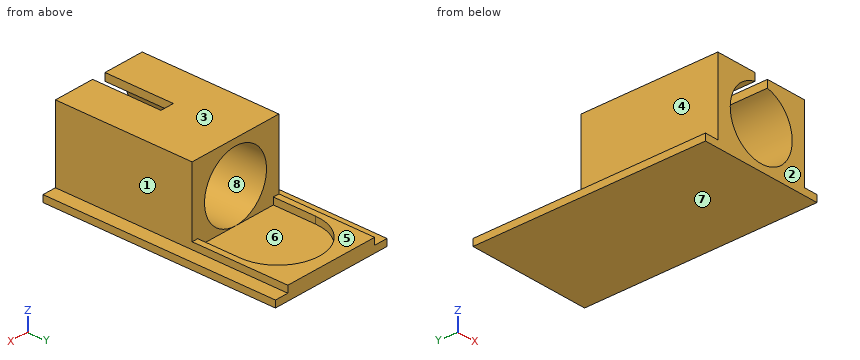
```python
from build123d import *

# Parameters (mm, degrees)
ESQUISSE1_W                  = 90
ESQUISSE1_H                  = 170
BOSS_EXTRU_1_DEPTH           = 5
ESQUISSE2_W                  = 70
ESQUISSE2_H                  = 100
BOSS_EXTRU_2_DEPTH           = 55
ENL_V_MAT_EXTRU_2_REACH      = 766.465
ESQUISSE4_R                  = 25
ENL_V_MAT_EXTRU_3_REACH      = 1014.096
ENL_V_MAT_EXTRU_3_END_RADIUS = 25
ESQUISSE5_W                  = 10
ESQUISSE5_H                  = 50
ESQUISSE6_W                  = 70
ESQUISSE6_H                  = 70
BOSS_EXTRU_3_DEPTH           = 5
ENL_V_MAT_EXTRU_4_DEPTH      = 5


with BuildPart() as part:
    # Esquisse1 → Boss.-Extru.1 (new body)
    with BuildSketch(Plane.XY):
        with Locations((-710.517990966, -585.769230769)):
            Rectangle(ESQUISSE1_W, ESQUISSE1_H)
    extrude(amount=BOSS_EXTRU_1_DEPTH)

    # Esquisse2 → Boss.-Extru.2 (add)
    with BuildSketch(Plane.XY.offset(5)):
        with Locations((-710.517990966, -620.769230769)):
            Rectangle(ESQUISSE2_W, ESQUISSE2_H)
    extrude(amount=BOSS_EXTRU_2_DEPTH)

    # Esquisse4 → Enlèv. mat.-Extru.2 (cut, up to next)
    with BuildSketch(Plane(origin=(0, -570.769230769, 0), x_dir=(1, 0, 0), z_dir=(0, 1, 0)), mode=Mode.PRIVATE) as enl_v_mat_extru_2_sk1:
        with Locations(Location((-710.517990966, -30, 0), (0, 0, 270))):
            Circle(ESQUISSE4_R)
    enl_v_mat_extru_2_tool1 = extrude(enl_v_mat_extru_2_sk1.sketch, amount=-ENL_V_MAT_EXTRU_2_REACH, mode=Mode.PRIVATE) & part.part
    add(enl_v_mat_extru_2_tool1.solids().sort_by_distance((-710.517991, -570.769231, 30))[0], mode=Mode.SUBTRACT)

    # Enlèv. mat.-Extru.3: up to this cylinder (the profile starts outside it)
    enl_v_mat_extru_3_end = Plane(origin=(-710.517990966, -645.769231, 30), z_dir=(0, 1, 0)) * Cylinder(ENL_V_MAT_EXTRU_3_END_RADIUS, 2079.192, mode=Mode.PRIVATE)
    # Esquisse5 → Enlèv. mat.-Extru.3 (cut, up to the surface)
    with BuildSketch(Plane.XY.offset(60), mode=Mode.PRIVATE) as enl_v_mat_extru_3_sk1:
        with Locations((-710.517990966, -645.769230769)):
            Rectangle(ESQUISSE5_W, ESQUISSE5_H)
    enl_v_mat_extru_3_tool1 = extrude(enl_v_mat_extru_3_sk1.sketch, amount=-ENL_V_MAT_EXTRU_3_REACH, mode=Mode.PRIVATE) - enl_v_mat_extru_3_end
    add(enl_v_mat_extru_3_tool1.solids().sort_by_distance((-710.517991, -645.769231, 60))[0], mode=Mode.SUBTRACT)

    # Esquisse6 → Boss.-Extru.3 (add)
    with BuildSketch(Plane.XY.offset(5)):
        with Locations((-710.517990966, -535.769230769)):
            Rectangle(ESQUISSE6_W, ESQUISSE6_H)
    extrude(amount=BOSS_EXTRU_3_DEPTH)

    # Esquisse7 → Enlèv. mat.-Extru.4 (cut)
    with BuildSketch(Plane.XY.offset(10)):
        with BuildLine():
            Line((-741.017990966, -539.769230769), (-741.017990966, -570.769230769))
            Line((-741.017990966, -570.769230769), (-680.017990966, -570.769230769))
            Line((-680.017990966, -570.769230769), (-680.017990966, -539.769230769))
            ThreePointArc((-680.017990966, -539.769230769), (-710.517990966, -509.269230769), (-741.017990966, -539.769230769))
        make_face()
    extrude(amount=-ENL_V_MAT_EXTRU_4_DEPTH, mode=Mode.SUBTRACT)


solid = part.part
```
Geometry check sheet. Reference: the model listing, model coordinates, mm. Face numbers are marked on the shaded views. A direction names the side the tool comes from. Coordinates: 2 decimals unless noted, no trailing zeros. Write each loop counter-clockwise with the first axis right and the second up, starting at its lowest first coordinate (ties: lowest second). Pieces come first, ordered by that corner, then holes. Notation, with made-up numbers: M -18.5,13.5 L -10.5,13.5 A13 cw -10.5,19.5 Z; hole C -4.75,25.5 d6. An arc over 180 degrees is marked long. Answer as a JSON object with one key per item and string values.
1. Scan lines: L1, parallel to X at y = -645, z = 30; L2, parallel to Y at x = -738.5, z = 50; L3, parallel to Y at x = -711, z = 8.5. Record each from-to range of solid material in increasing order.
Answers below:
{"L1": "x = -745.52 to -735.52, -685.52 to -675.52", "L2": "y = -670.77 to -570.77", "L3": "y = -509.27 to -500.77"}
2. Section check C-C, the plane y = -538. Enter the section's corners in (x, z).
Answers below:
{"outline": "M -755.52,0 L -665.52,0 L -665.52,5 L -675.52,5 L -675.52,10 L -680.07,10 L -680.07,5 L -740.97,5 L -740.97,10 L -745.52,10 L -745.52,5 L -755.52,5 Z"}
3. Section check B-B, the plane x = -700. Enter the section's corners in (y, z), plus the area to 3 significant figures.
Answers below:
{"outline": "M -670.77,0 L -500.77,0 L -500.77,10 L -511.14,10 L -511.14,5 L -570.77,5 L -570.77,7.32 L -670.77,7.32 Z; M -670.77,52.68 L -570.77,52.68 L -570.77,60 L -670.77,60 Z", "area": "1,870 mm²"}
4. Section check D-D, the plane x = -712.5. Enter the section's corners in (y, z).
Answers below:
{"outline": "M -670.77,0 L -500.77,0 L -500.77,10 L -509.33,10 L -509.33,5 L -570.77,5 L -570.77,5.08 L -670.77,5.08 Z; M -620.77,54.92 L -570.77,54.92 L -570.77,60 L -620.77,60 Z"}
5. Tool access check on the marked faces 1, 2, 3, 4 and 5. Record the directions out of +Z, -Z, +X, -X, +Y, -Y that give a thin tool (end or side, any length) a straight path to the whole face; none if there is none.
Answers below:
{"face 1": "+Z, +X, +Y, -Y", "face 2": "+Z, -Z, +X, -X, -Y", "face 3": "+Z, +X, -X, +Y, -Y", "face 4": "+Z, -X, +Y, -Y", "face 5": "+Z, +X, -X, +Y"}
6. Go/stop test with flat-tipped pins: pin 1 Ø4 at (y, z) = (-549, 7.5) entering from -X; pin 2 Ø1 at (y, z) = (-567.5, 9.5) entering from +X; pin 3 Ø5 at (x, y) = (-752, -614.5) entering from +Z. Record where each tip stops, or that it passes through.
Answers below:
{"pin 1": "stops at x = -745.52", "pin 2": "stops at x = -675.52", "pin 3": "stops at z = 5"}
7. Draft check along Z on the marked faces 6, 7 and 8. Enter one of: released by +Z, released by -Z, zero draft, split by the parting line, or undercut.
Answers below:
{"face 6": "released by +Z", "face 7": "released by -Z", "face 8": "undercut"}
8. Section check A-A, the plane z = 30. Enter the section's corners in (x, y).
Answers below:
{"outline": "M -745.52,-670.77 L -735.52,-670.77 L -735.52,-570.77 L -745.52,-570.77 Z; M -685.52,-670.77 L -675.52,-670.77 L -675.52,-570.77 L -685.52,-570.77 Z"}
